The listing builds one solid part. Answer for the finished solid, in the listing's coordinates (mm). Round coordinates to 2 decimals unless told otherwise and drop trailing zeros. Loops run counter-clockwise (first coordinate to the right, second up) from the corner with the lowest first, then second, coordinate; pieces in that order, holes last. Notation, with made-up numbers: (1.5, 54) -> (50.5, 54) arc R21 ccw to (50.5, 79) -> close; hole circle Ø3 at (10.5, 77.25). An arc over 180 degrees is marked (long way). Write each question's results on one line, items separated by ' | '. Start each with the question number.
(1) A flat-ended cylindrical pin translates along its axis: pin 1 (0.7 mm diameter, centred on x = -4, z = -2.5, fed in from -Y). Find the tip coordinate at first contact, or state that the pin passes through.
(2) Straight lines are drawn through the part: probe 1 along Y at (x, z) = (-3, -2.7); probe 2 along Y at (x, z) = (-4.5, -4.05). For each, find the intervals that lie inside material, in ascending order.
(3) The part is cut by section A-A (y = 19.05). Determine the outline of the cut face in (x, z), plus the area to 3 significant figures.
Autodesk Inventor part; units mm, degrees
ref_plane "YZ Plane" through (0, 0, 0) normal (1, 0, 0) x (0, 1, 0)
ref_plane "XZ Plane" through (0, 0, 0) normal (0, 1, 0) x (-1, 0, 0)
ref_plane "XY Plane" through (0, 0, 0) normal (0, 0, 1) x (1, 0, 0)
sketch "Sketch1" plane through (0, 0, 0) normal (0, 1, 0) x (-1, 0, 0)
  line L0 (0, 0) -> (6.35, 0)
  line L1 (6.35, 0) -> (6.35, -4.7625)
  line L2 (6.35, -4.7625) -> (0, -4.7625)
  line L3 (0, -4.7625) -> (0, 0)
  circle A0 centre (3.175, -2.3812) radius 1.7526
  dimension "d0" = 6.35
  dimension "d1" = 4.7625
  dimension "d2" = 3.5052
extrude "Extrusion1" add sketch "Sketch1" along normal blind 176.182 contours L0 L1 L2 L3 | A0
sketch "Sketch2" plane through (-6.35, 0, 0) normal (0, 0, 1) x (1, 0, 0)
  line L0 (6.35, 176.182) -> (0, 176.182)
  line L1 (3.175, 176.182) -> (3.175, 173.007)
  circle A0 centre (3.175, 173.007) radius 1.7526
  line L2 (6.35, 0) -> (0, 0)
  line L3 (3.175, 0) -> (3.175, 19.05)
  circle A1 centre (3.175, 19.05) radius 1.7526
  line L4 (3.175, 0) -> (3.175, 12.7)
  circle A2 centre (3.175, 12.7) radius 0.508
  line L5 (3.175, 173.007) -> (3.175, 73.007)
  circle A3 centre (3.175, 73.007) radius 1.7526
  dimension "d5" = 3.175
  dimension "d6" = 3.5052
  dimension "d14" = 19.05
  dimension "d15" = 3.5052
  dimension "d16" = 12.7
  dimension "d17" = 1.016
  dimension "d47" = 100.0001
  dimension "d48" = 3.5052
hole "Hole2" at (-3.175, 19.05, 0) direction (0, 0, -1) diameter 3.7973 end through all
hole "Hole3" at (-3.175, 12.7, 0) direction (0, 0, -1) diameter 1.016 end through all
hole "Hole4" at (-3.175, 173.007, 0) direction (0, 0, -1) diameter 3.7973 end through all
sketch "Sketch3" plane through (0, 0, 0) normal (0, -1, 0) x (1, 0, 0)
  line L0 (0, -4.7625) -> (-6.35, -4.7625)
  line L1 (-6.35, -4.7625) -> (0, 0)
  circle A0 centre (-3.175, -2.3812) radius 1.3208
  dimension "d39" = 2.6416
hole "Hole5" at (-3.175, 0, -2.3812) direction (0, 1, 0) diameter 2.6416 depth 12.7
hole "Hole6" at (-3.175, 73.007, 0) direction (0, 0, -1) diameter 3.7973 end through all
properties part number "rod(6-32)"
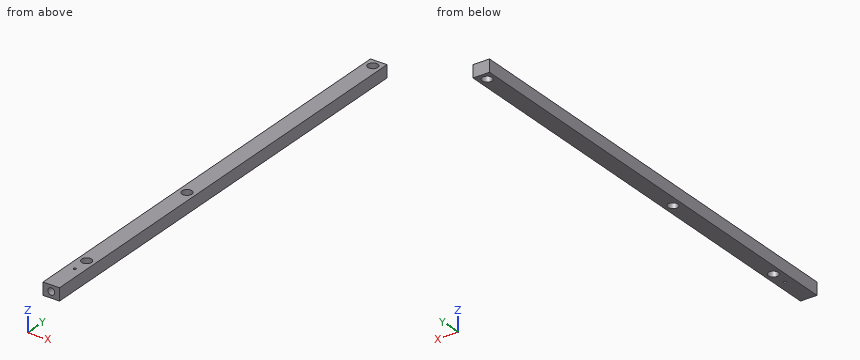
Checked values:
1) pin 1: stops at y = 12.7
2) probe 1: y = 13.18 to 17.16, 20.94 to 71.12, 74.9 to 171.12, 174.9 to 176.18 | probe 2: y = 0 to 17.69, 20.41 to 71.65, 74.37 to 171.65, 174.37 to 176.18
3) outline: (-6.35, -4.76) -> (-5.07, -4.76) -> (-5.07, 0) -> (-6.35, 0) -> close; (-1.28, -4.76) -> (0, -4.76) -> (0, 0) -> (-1.28, 0) -> close | area: 12.2 mm2
